Design review of the part built by this model. Coordinates are the model's own, in mm. Round coordinates to 2 decimals unless told otherwise and drop trailing zeros. Loops run counter-clockwise (first coordinate to the right, second up) from the corner with the lowest first, then second, coordinate; pieces in that order, holes last. Notation, with made-up numbers: (36, -39.5) -> (67, -39.5) arc R21 cw to (67, -31.5) -> close; hole circle Ø10 at (56, -20.5). An arc over 180 degrees is marked (long way). Use a Markdown table: item, result. Add a question column.
Autodesk Inventor part; units mm, degrees
ref_plane "YZ Plane" through (0, 0, 0) normal (1, 0, 0) x (0, 1, 0)
ref_plane "XZ Plane" through (0, 0, 0) normal (0, 1, 0) x (-1, 0, 0)
ref_plane "XY Plane" through (0, 0, 0) normal (0, 0, 1) x (1, 0, 0)
sketch "Skizze1" plane through (0, 0, 0) normal (1, 0, 0) x (0, 1, 0)
  line L0 (0, -30.1) -> (0, 30.1)
  line L1 (-45.5, 0) -> (45.5, 0)
  line L2 (-30.5, 21.5) -> (30.5, 21.5)
  line L3 (32.5, 19.5) -> (32.5, -19.5)
  line L4 (30.5, -21.5) -> (-30.5, -21.5)
  line L5 (-32.5, -19.5) -> (-32.5, 19.5)
  circle A0 centre (22.5, 13.5) radius 2.75
  circle A1 centre (22.5, -13.5) radius 2.75
  line L6 (30.5, 21.5) -> (32.5, 19.5)
  line L7 (32.5, -19.5) -> (30.5, -21.5)
  line L8 (-30.5, 21.5) -> (-32.5, 19.5)
  line L9 (-30.5, -21.5) -> (-32.5, -19.5)
  circle A2 centre (-11, 0) radius 12
  circle A3 centre (-26.5, 15.5) radius 1.75
  circle A4 centre (-26.5, -15.5) radius 1.75
  circle A5 centre (4.5, 15.5) radius 1.75
  circle A6 centre (4.5, -15.5) radius 1.75
  point P0 (0, 0)
  point P1 (-32.5, 21.5)
  point P2 (32.5, -21.5)
  point P3 (32.5, 21.5)
  point P4 (-32.5, -21.5)
  dimension "d0" = 65
  dimension "d1" = 43
  dimension "d2" = 5.5
  dimension "d3" = 10
  dimension "d4" = 8
  dimension "d14" = 2
  dimension "d15" = 2
  dimension "d16" = 2
  dimension "d17" = 2
  dimension "d18" = 2
  dimension "d19" = 2
  dimension "d20" = 2
  dimension "d21" = 2
  dimension "d35" = 24
  dimension "d43" = 3.5
  dimension "d44" = 15.5
  dimension "d46" = 15.5
  dimension "d47" = 21.5
  dimension "d48" = 3.5
  dimension "d49" = 15.5
  dimension "d50" = 15.5
extrude "Extrusion5" add sketch "Skizze1" along normal blind 3 contours L4 L9 L5 L1 A2 L0 | L0 A2 L1 L3 L7 L4 | L1 L5 L8 L2 L0 A2 | A2 L0 L2 L6 L3 L1
properties part number "Nema17_Montageplatte_Extruder" material "Aluminium 6061"
1. Consider section B-B on z = 0. State the section outline as (x, y) points.
2. Consider section D-D on y = -11. State the section outline as (x, z) points, plus the area to 3 significant figures.
3. Consider section A-A on y = -26.5. State the section outline as (x, z) points, plus the area to 3 significant figures.
4. To check wall thickness, follow probe 1 along Z at (x, y) = (2.2, 4.5); probe 2 along Z at (x, y) = (1.2, 6); probe 3 along Y at (x, z) = (0.7, -15). State the ranges of each line that lie inside material, in increasing order. Write a range as from..to.
5. Consider section C-C on x = 1.4. State the section outline as (y, z) points.
6. Insertion check: P1, Ø3, axis at y = -26.5, z = 15.5, coming from the -X side. The pin has a flat end and moves straight along its axis. Give the tip position at first contact, or say it passes through.
7. Mouldability with a two-part tool opening along Z and no side actions: class faces 1 (the face through (1, 31, 21)), 2 (the face through (1.479, 19.753, -13.621)), 3 (the face through (3, 7, 0)) as +Z half, -Z half, draft (parallel to the pull), parting line (faces both ways), or undercut.
Verdict:
| question | item | result |
|---|---|---|
| 1 | outline | (0, -32.5) -> (3, -32.5) -> (3, -23) -> (0, -23) -> close; (0, 1) -> (3, 1) -> (3, 32.5) -> (0, 32.5) -> close |
| 2 | outline | (0, -21.5) -> (3, -21.5) -> (3, -12) -> (0, -12) -> close; (0, 12) -> (3, 12) -> (3, 21.5) -> (0, 21.5) -> close |
| 2 | area | 57.0 mm² |
| 3 | outline | (0, -21.5) -> (3, -21.5) -> (3, -17.25) -> (0, -17.25) -> close; (0, -13.75) -> (3, -13.75) -> (3, 13.75) -> (0, 13.75) -> close; (0, 17.25) -> (3, 17.25) -> (3, 21.5) -> (0, 21.5) -> close |
| 3 | area | 108 mm² |
| 4 | probe 1 | z = -21.5..-17.25, -13.75..13.75, 17.25..21.5 |
| 4 | probe 2 | z = -21.5..-16.4, -14.6..14.6, 16.4..21.5 |
| 4 | probe 3 | y = -32.5..-28.18, -24.82..2.82, 6.18..20.2, 24.8..32.5 |
| 5 | outline | (-32.5, -19.5) -> (-30.5, -21.5) -> (30.5, -21.5) -> (32.5, -19.5) -> (32.5, 19.5) -> (30.5, 21.5) -> (-30.5, 21.5) -> (-32.5, 19.5) -> close; hole circle Ø3.5 at (-26.5, -15.5); hole circle Ø3.5 at (-26.5, 15.5); hole circle Ø24 at (-11, 0); hole circle Ø3.5 at (4.5, -15.5); hole circle Ø3.5 at (4.5, 15.5); hole circle Ø5.5 at (22.5, -13.5); hole circle Ø5.5 at (22.5, 13.5) |
| 6 | P1 | passes through |
| 7 | face 1 | +Z half |
| 7 | face 2 | undercut |
| 7 | face 3 | draft |
